Verification items for the finished model (mm, model axes). Round coordinates to 2 decimals unless told otherwise and drop trailing zeros. Write each loop counter-clockwise with the first axis right and the second up, starting at its lowest first coordinate (ties: lowest second). Pieces come first, ordered by that corner, then holes. Notation, with made-up numbers: M 83.5,30 L 95.5,30 A20 ccw 95.5,42 Z; hole C 86,75.25 d5. An arc over 180 degrees is marked long. One line per question, with ' | ' between items. Start each with the question number.
Q1. Cross-section at B-B (y = 0.5). Record the boundary of the cut face in (x, z).
Q2. Thickness scan on line 1 along Y through (x, z) = (44, 6); line 2 along X through (y, z) = (245, 1); line 3 along Y through (x, z) = (436, 4.75). Record the ranges inside material, lowest first. Write a range as from..to.
Q3. Gauge pin test, flat end, axial feed: pin 1 (1.5 mm diameter, centred on x = 653, z = 4.5, fed in from +Y). Record the tip position at first contact, or that the pin passes through.
Q4. Cross-section at A-A (x = 192.5). Record the boundary of the cut face in (y, z).
from build123d import *

# Parameters (mm, degrees)
BOSS_EXTRUDE1_DEPTH = 6.35


with BuildPart() as part:
    # Sketch1 → Boss-Extrude1 (new body)
    with BuildSketch(Plane.XY):
        with BuildLine():
            Line((4.79079833, -60.96), (439.701599067, -60.96))
            ThreePointArc((439.701599067, -60.96), (565.425184762, -8.883585695), (617.501599067, 116.84))
            add(Edge.make_bspline(
                [(617.501599067, 116.84), (617.501599067, 198.103261629), (630.412866299, 310.67677722), (736.575869498, 358.14), (821.560436263, 358.14)],
                knots=[0, 0, 0, 0, 0.504521354, 1, 1, 1, 1], degree=3))
            Line((821.560436263, 358.14), (821.560436263, 408.94))
            Line((821.560436263, 408.94), (726.691494057, 408.94))
            ThreePointArc((726.691494057, 408.94), (637.145879185, 379.858055682), (581.775600083, 303.711428571))
            ThreePointArc((581.775600083, 303.711428571), (443.349902326, 113.344860795), (219.485865145, 40.64))
            Line((219.485865145, 40.64), (4.79079833, 40.64))
            ThreePointArc((4.79079833, 40.64), (-13.169713912, 33.200512242), (-20.60920167, 15.24))
            Line((-20.60920167, 15.24), (-20.60920167, -35.56))
            ThreePointArc((-20.60920167, -35.56), (-13.169713912, -53.520512242), (4.79079833, -60.96))
        make_face()
    extrude(amount=BOSS_EXTRUDE1_DEPTH)


solid = part.part
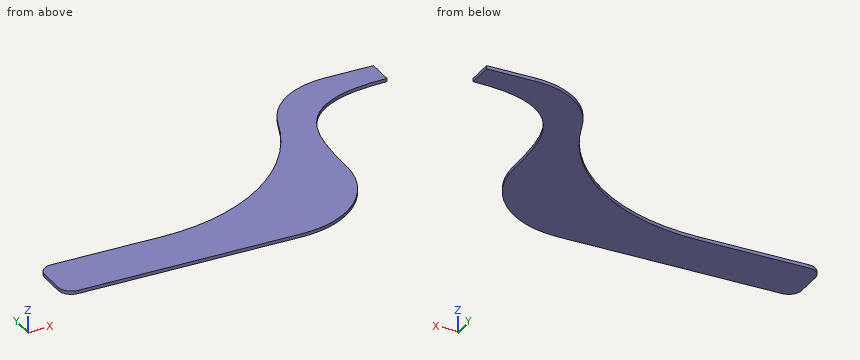
Determined:
1) outline: M -20.61,0 L 574.16,0 L 574.16,6.35 L -20.61,6.35 Z
2) line 1: y = -60.96..40.64 | line 2: x = 557.06..630.06 | line 3: y = -60.96..108.14
3) pin 1: stops at y = 390.35
4) outline: M -60.96,0 L 40.64,0 L 40.64,6.35 L -60.96,6.35 Z
